```python
from build123d import *

# Parameters (mm, degrees)
F0_R     = 8.5
F1_DEPTH = 30
F0_R_2   = 14
F2_DEPTH = 5
F0_R_3   = 16
F3_DEPTH = 10
F4_R     = 4
F5_R     = 6


with BuildPart() as f1:
    # F0 (on Top) → F1 (new body)
    with BuildSketch(Plane.XY):
        Circle(F0_R)
    extrude(amount=F1_DEPTH)

    # F0 (on Top) → F2 (join)
    with BuildSketch(Plane.XY):
        Circle(F0_R_2)
        Circle(F0_R, mode=Mode.SUBTRACT)
    extrude(amount=F2_DEPTH)

    # F0 (on Top) → F3 (join)
    with BuildSketch(Plane.XY):
        Circle(F0_R_3)
        Circle(F0_R_2, mode=Mode.SUBTRACT)
    extrude(amount=F3_DEPTH)

    # F4
    f4_edges = [f1.edges().sort_by_distance(p)[0] for p in [
        (-8.5, 0, 30),
    ]]
    fillet(f4_edges, radius=F4_R)

    # F5
    f5_edges = [f1.edges().sort_by_distance(p)[0] for p in [
        (-16, 0, 0),
    ]]
    fillet(f5_edges, radius=F5_R)


solid = f1.part
```
For this review, take the finished solid that the model builds, in its own axes (mm). A direction names the side the tool comes from. Round coordinates to 2 decimals unless told otherwise and drop trailing zeros. Write each loop counter-clockwise with the first axis right and the second up, starting at its lowest first coordinate (ties: lowest second). Pieces come first, ordered by that corner, then holes. Notation, with made-up numbers: (-37, 62.5) -> (-20, 62.5) arc R27 cw to (-20, 82.5) -> close; hole circle Ø5 at (79, 42). An arc over 180 degrees is marked (long way). Use one line per item in the form item = value.
Q1. Consider section D-D (z = 3.5). State the section outline as (x, y) points, then the cut area to 3 significant figures.
Resolved:
outline = circle Ø30.91 at (0, 0)
area = 750 mm²
Q2. To check wall thickness, follow probe 1 along Y at (x, z) = (0, 9.5); probe 2 along X at (y, z) = (-3.5, 6.75); probe 3 along Z at (x, y) = (-2, -10). State the ranges of each line that lie inside material, in increasing order. Write a range as from..to.
Resolved:
probe_1 = -16..-14, -8.5..8.5, 14..16
probe_2 = -15.61..-13.56, -7.75..7.75, 13.56..15.61
probe_3 = 0..5
Q3. The part is to be moulded in two halves that separate along X. For faces 1 (the flat face through (0, -9, 5)), 2 (the flat face through (0, 0, 0)), 3 (the cylindrical face through (-3.47, -15.62, 7.97)), say which applies: released by +X, released by -X, zero draft, split by the parting line, or undercut.
Resolved:
face_1 = undercut
face_2 = zero draft
face_3 = split by the parting line
Q4. Clearance check with flat-ended pins moving along their axes: pin 1 Ø4 at (x, z) = (-9.5, 19) entering from +Y; pin 2 Ø1.5 at (x, y) = (-6, 11) entering from +Z; pin 3 Ø2 at (y, z) = (-4.5, 7.5) entering from +X. State where each tip first meets the part, or that it passes through.
Resolved:
pin_1 = 4
pin_2 = 5
pin_3 = 15.61
Q5. Consider section A-A (y = 0). State the section outline as (x, z) points, then the cut area to 3 significant figures.
Resolved:
outline = (-16, 6) arc R6 ccw to (-10, 0) -> (10, 0) arc R6 ccw to (16, 6) -> (16, 10) -> (14, 10) -> (14, 5) -> (8.5, 5) -> (8.5, 26) arc R4 ccw to (4.5, 30) -> (-4.5, 30) arc R4 ccw to (-8.5, 26) -> (-8.5, 5) -> (-14, 5) -> (-14, 10) -> (-16, 10) -> close
area = 583 mm²
Q6. Consider section C-C (z = 23.5). State the section outline as (x, y) points, then the cut area to 3 significant figures.
Resolved:
outline = circle Ø17 at (0, 0)
area = 227 mm²
Q7. Machinability: for faces 4 (the cylindrical face through (12.932, -5.362, 7.465)), 5 (the flat face through (0, 0, 30)), which of the approach directions +Z, -Z, +X, -X, +Y, -Y give a long, thin tool a straight path to every point of the face, cutting with its end or side? Answer none if there is none.
Resolved:
face_4 = +Z
face_5 = +Z, +X, -X, +Y, -Y
